Input: part model. Units: mm. Frame: model coordinates. Round coordinates to 2 decimals unless told otherwise and drop trailing zeros. Loops run counter-clockwise (first coordinate to the right, second up) from the corner with the lowest first, then second, coordinate; pieces in that order, holes last. Notation, with made-up numbers: (-19.5, 23) -> (15.5, 23) arc R7 ccw to (15.5, 28) -> close; hole circle Ø3 at (18.5, -26.75). An arc over 180 degrees is marked (long way). Answer in a Markdown table with one row per item. Add a question column.
Q1. Pin query (flat end, axial travel): pin 1 (2 mm diameter, centred on y = -2.5, z = 2, fed in from +X); pin 2 (1.5 mm diameter, centred on x = -15.5, z = 2.5, fed in from +Y); pin 3 (1 mm diameter, centred on x = 5.5, z = 1, fed in from -Y). Return the tip coordinate at first contact, or that it passes through.
Q2. Section B-B, the plane x = 4. Output: boundary loops of the cut face in (y, z), and give its area (3 significant figures).
Q3. Section A-A, the plane z = 4.3. Give the number of separate pieces and of enclosed holes in the cut face, and give its area (3 significant figures).
Q4. Section C-C, the plane x = -8.5. Output: boundary loops of the cut face in (y, z).
Q5. Ray query, L1, parallel to Y at x = -16.5, z = 1.5; L2, parallel to Y at x = 14.5, z = 4.1; L3, parallel to Y at x = 11.5, z = 3. Return the intervals inside material, ascending. Write a range as from..to.
```python
from build123d import *

# Parameters (mm, degrees)
SKETCH1_R           = 1.5
BOSS_EXTRUDE1_DEPTH = 5


with BuildPart() as part:
    # Sketch1 → Boss-Extrude1 (new body)
    with BuildSketch(Plane.XY):
        with BuildLine():
            Line((3.341817931, 17.286797691), (4.939453025, 18.264687321))
            ThreePointArc((4.939453025, 18.264687321), (6.271018689, 18.696765153), (7.653668647, 18.47759065))
            ThreePointArc((7.653668647, 18.47759065), (8.86205197, 17.562621273), (9.468927016, 16.173714546))
            Line((9.468927016, 16.173714546), (9.702808263, 14.692060213))
            Line((9.702808263, 14.692060213), (11.553052787, 14.984123946))
            ThreePointArc((11.553052787, 14.984123946), (12.948608078, 14.873743692), (14.142135624, 14.142135624))
            ThreePointArc((14.142135624, 14.142135624), (14.908392622, 12.834385865), (14.937560462, 11.318962342))
            Line((14.937560462, 11.318962342), (14.586633993, 9.860589752))
            Line((14.586633993, 9.860589752), (16.407804991, 9.422363532))
            ThreePointArc((16.407804991, 9.422363532), (17.654889266, 8.786329586), (18.47759065, 7.653668647))
            ThreePointArc((18.47759065, 7.653668647), (18.685065641, 6.152231554), (18.132085736, 4.741000729))
            Line((18.132085736, 4.741000729), (17.249776925, 3.527933887))
            Line((17.249776925, 3.527933887), (18.764617622, 2.426133683))
            ThreePointArc((18.764617622, 2.426133683), (19.673373605, 1.361276448), (20, 0))
            ThreePointArc((20, 0), (19.617106797, -1.466544242), (18.566165325, -2.558735269))
            Line((18.566165325, -2.558735269), (17.286797691, -3.341817931))
            Line((17.286797691, -3.341817931), (18.264687321, -4.939453025))
            ThreePointArc((18.264687321, -4.939453025), (18.696765153, -6.271018689), (18.47759065, -7.653668647))
            ThreePointArc((18.47759065, -7.653668647), (17.562621273, -8.86205197), (16.173714546, -9.468927016))
            Line((16.173714546, -9.468927016), (14.692060213, -9.702808263))
            Line((14.692060213, -9.702808263), (14.984123946, -11.553052787))
            ThreePointArc((14.984123946, -11.553052787), (14.873743692, -12.948608078), (14.142135624, -14.142135624))
            ThreePointArc((14.142135624, -14.142135624), (12.834385865, -14.908392622), (11.318962342, -14.937560462))
            Line((11.318962342, -14.937560462), (9.860589752, -14.586633993))
            Line((9.860589752, -14.586633993), (9.422363532, -16.407804991))
            ThreePointArc((9.422363532, -16.407804991), (8.786329586, -17.654889266), (7.653668647, -18.47759065))
            ThreePointArc((7.653668647, -18.47759065), (6.152231554, -18.685065641), (4.741000729, -18.132085736))
            Line((4.741000729, -18.132085736), (3.527933887, -17.249776925))
            Line((3.527933887, -17.249776925), (2.426133683, -18.764617622))
            ThreePointArc((2.426133683, -18.764617622), (1.361276448, -19.673373605), (0, -20))
            ThreePointArc((0, -20), (-1.466544242, -19.617106797), (-2.558735269, -18.566165325))
            Line((-2.558735269, -18.566165325), (-3.341817931, -17.286797691))
            Line((-3.341817931, -17.286797691), (-4.939453025, -18.264687321))
            ThreePointArc((-4.939453025, -18.264687321), (-6.271018689, -18.696765153), (-7.653668647, -18.47759065))
            ThreePointArc((-7.653668647, -18.47759065), (-8.86205197, -17.562621273), (-9.468927016, -16.173714546))
            Line((-9.468927016, -16.173714546), (-9.702808263, -14.692060213))
            Line((-9.702808263, -14.692060213), (-11.553052787, -14.984123946))
            ThreePointArc((-11.553052787, -14.984123946), (-12.948608078, -14.873743692), (-14.142135624, -14.142135624))
            ThreePointArc((-14.142135624, -14.142135624), (-14.908392622, -12.834385865), (-14.937560462, -11.318962342))
            Line((-14.937560462, -11.318962342), (-14.586633993, -9.860589752))
            Line((-14.586633993, -9.860589752), (-16.407804991, -9.422363532))
            ThreePointArc((-16.407804991, -9.422363532), (-17.654889266, -8.786329586), (-18.47759065, -7.653668647))
            ThreePointArc((-18.47759065, -7.653668647), (-18.685065641, -6.152231554), (-18.132085736, -4.741000729))
            Line((-18.132085736, -4.741000729), (-17.249776925, -3.527933887))
            Line((-17.249776925, -3.527933887), (-18.764617622, -2.426133683))
            ThreePointArc((-18.764617622, -2.426133683), (-19.673373605, -1.361276448), (-20, 0))
            ThreePointArc((-20, 0), (-19.617106797, 1.466544242), (-18.566165325, 2.558735269))
            Line((-18.566165325, 2.558735269), (-17.286797691, 3.341817931))
            Line((-17.286797691, 3.341817931), (-18.264687321, 4.939453025))
            ThreePointArc((-18.264687321, 4.939453025), (-18.696765153, 6.271018689), (-18.47759065, 7.653668647))
            ThreePointArc((-18.47759065, 7.653668647), (-17.562621273, 8.86205197), (-16.173714546, 9.468927016))
            Line((-16.173714546, 9.468927016), (-14.692060213, 9.702808263))
            Line((-14.692060213, 9.702808263), (-14.984123946, 11.553052787))
            ThreePointArc((-14.984123946, 11.553052787), (-14.873743692, 12.948608078), (-14.142135624, 14.142135624))
            ThreePointArc((-14.142135624, 14.142135624), (-12.834385865, 14.908392622), (-11.318962342, 14.937560462))
            Line((-11.318962342, 14.937560462), (-9.860589752, 14.586633993))
            Line((-9.860589752, 14.586633993), (-9.422363532, 16.407804991))
            ThreePointArc((-9.422363532, 16.407804991), (-8.786329586, 17.654889266), (-7.653668647, 18.47759065))
            ThreePointArc((-7.653668647, 18.47759065), (-6.152231554, 18.685065641), (-4.741000729, 18.132085736))
            Line((-4.741000729, 18.132085736), (-3.527933887, 17.249776925))
            Line((-3.527933887, 17.249776925), (-2.426133683, 18.764617622))
            ThreePointArc((-2.426133683, 18.764617622), (-1.361276448, 19.673373605), (0, 20))
            ThreePointArc((0, 20), (1.466544242, 19.617106797), (2.558735269, 18.566165325))
            Line((2.558735269, 18.566165325), (3.341817931, 17.286797691))
        make_face()
        with Locations((0, 17)):
            Circle(SKETCH1_R, mode=Mode.SUBTRACT)
        with Locations((6.50561835, 15.705952053)):
            Circle(SKETCH1_R, mode=Mode.SUBTRACT)
        with Locations((12.02081528, 12.02081528)):
            Circle(SKETCH1_R, mode=Mode.SUBTRACT)
        with Locations((15.705952053, 6.50561835)):
            Circle(SKETCH1_R, mode=Mode.SUBTRACT)
        with Locations((17, 0)):
            Circle(SKETCH1_R, mode=Mode.SUBTRACT)
        with Locations((15.705952053, -6.50561835)):
            Circle(SKETCH1_R, mode=Mode.SUBTRACT)
        with Locations((12.02081528, -12.02081528)):
            Circle(SKETCH1_R, mode=Mode.SUBTRACT)
        with Locations((6.50561835, -15.705952053)):
            Circle(SKETCH1_R, mode=Mode.SUBTRACT)
        with Locations((0, -17)):
            Circle(SKETCH1_R, mode=Mode.SUBTRACT)
        with Locations((-6.50561835, -15.705952053)):
            Circle(SKETCH1_R, mode=Mode.SUBTRACT)
        with Locations((-12.02081528, -12.02081528)):
            Circle(SKETCH1_R, mode=Mode.SUBTRACT)
        with Locations((-15.705952053, -6.50561835)):
            Circle(SKETCH1_R, mode=Mode.SUBTRACT)
        with Locations((-17, 0)):
            Circle(SKETCH1_R, mode=Mode.SUBTRACT)
        with Locations((-15.705952053, 6.50561835)):
            Circle(SKETCH1_R, mode=Mode.SUBTRACT)
        with Locations((-12.02081528, 12.02081528)):
            Circle(SKETCH1_R, mode=Mode.SUBTRACT)
        with Locations((-6.50561835, 15.705952053)):
            Circle(SKETCH1_R, mode=Mode.SUBTRACT)
    extrude(amount=BOSS_EXTRUDE1_DEPTH)


solid = part.part
```
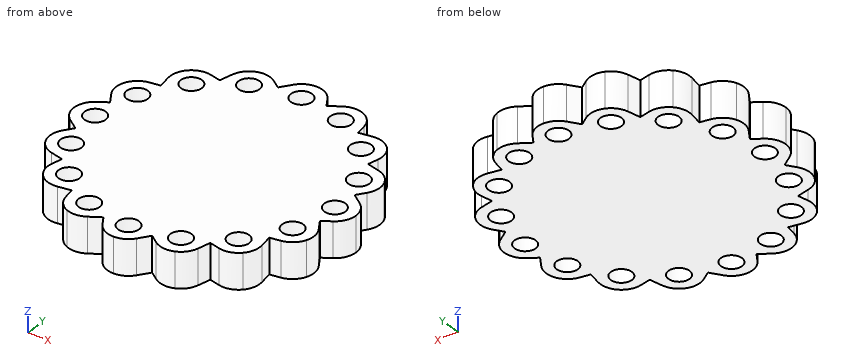
Answer block:
| question | item | result |
|---|---|---|
| 1 | pin 1 | x = 19.6 |
| 1 | pin 2 | y = 13.27 |
| 1 | pin 3 | y = -18.66 |
| 2 | outline | (-17.59, 0) -> (17.69, 0) -> (17.69, 5) -> (-17.59, 5) -> close |
| 2 | area | 176 mm^2 |
| 3 | separate pieces | 1 |
| 3 | enclosed holes | 16 |
| 3 | area | 1,040 mm^2 |
| 4 | outline | (-17.95, 0) -> (17.95, 0) -> (17.95, 5) -> (-17.95, 5) -> close |
| 5 | L1 | -9.4..-7.78, -5.23..-1.41, 1.41..5.23, 7.78..9.4 |
| 5 | L2 | -13.71..-7.4, -5.61..5.61, 7.4..13.71 |
| 5 | L3 | -14.98..-13.43, -10.61..10.61, 13.43..14.98 |
